Model file for the job. Use its own axes, mm. Face numbers are marked on the shaded views. A direction names the side the tool comes from. Round coordinates to 2 decimals unless told otherwise and drop trailing zeros. Loops run counter-clockwise (first coordinate to the right, second up) from the corner with the lowest first, then second, coordinate; pieces in that order, holes last. Notation, with made-up numbers: M 0.5,-27 L 29.5,-27 A20 cw 29.5,8 Z; hole C -24,-38.75 d10. An arc over 180 degrees is marked long. Answer in a Markdown table with one row per item.
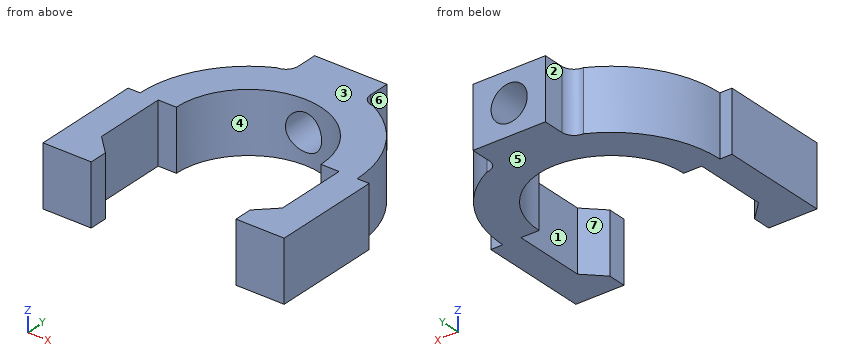
from build123d import *

# Parameters (mm, degrees)
BOSS_EXTRUDE1_DEPTH = 20
SKETCH2_R           = 6
CUT_EXTRUDE1_DEPTH  = 20


with BuildPart() as part:
    # Sketch1 → Boss-Extrude1 (new body)
    with BuildSketch(Plane.XY):
        with BuildLine():
            Line((0, 0), (0, -7))
            ThreePointArc((0, -7), (-1.171572875, -9.828427125), (-4, -11))
            ThreePointArc((-4, -11), (-18.594117082, -24.275365032), (-24, -43.249030993))
            Line((-24, -43.249030993), (-28, -43.249030993))
            Line((-28, -43.249030993), (-28, -79.249030993))
            Line((-28, -79.249030993), (-12, -79.249030993))
            Line((-12, -79.249030993), (-12, -73.249030993))
            Line((-12, -73.249030993), (-18, -67.249030993))
            Line((-18, -67.249030993), (-18, -43.249030993))
            Line((-18, -43.249030993), (-12, -43.249030993))
            ThreePointArc((-12, -43.249030993), (12, -19.249030993), (36, -43.249030993))
            Line((36, -43.249030993), (42, -43.249030993))
            Line((42, -43.249030993), (42, -67.249030993))
            Line((42, -67.249030993), (36, -73.249030993))
            Line((36, -73.249030993), (36, -79.249030993))
            Line((36, -79.249030993), (52, -79.249030993))
            Line((52, -79.249030993), (52, -43.249030993))
            Line((52, -43.249030993), (48, -43.249030993))
            ThreePointArc((48, -43.249030993), (42.594117082, -24.275365032), (28, -11))
            ThreePointArc((28, -11), (25.171572875, -9.828427125), (24, -7))
            Line((24, -7), (24, 0))
            Line((24, 0), (0, 0))
        make_face()
    extrude(amount=BOSS_EXTRUDE1_DEPTH)

    # Sketch2 → Cut-Extrude1 (cut)
    with BuildSketch(Plane(origin=(0, 0, 0), x_dir=(1, 0, 0), z_dir=(0, 1, 0))):
        with Locations((12, -10)):
            Circle(SKETCH2_R)
    extrude(amount=-CUT_EXTRUDE1_DEPTH, mode=Mode.SUBTRACT)


solid = part.part
1. Saw through at B-B (x = 12). Write the cut outline in (y, z), and give its area (3 significant figures).
Verdict:
| item | result |
|---|---|
| outline | M -19.25,0 L 0,0 L 0,4 L -19.25,4 Z; M -19.25,16 L 0,16 L 0,20 L -19.25,20 Z |
| area | 154 mm² |
2. Saw through at C-C (y = -17). Write the cut outline in (x, z).
Verdict:
| item | result |
|---|---|
| outline | M -12.64,0 L 36.64,0 L 36.64,20 L -12.64,20 Z; hole C 12,10 d12 |
3. Mould opens along X. For the marked faces 1, 2, 3 and 4 say: +X half, -X half, draft (parallel to the pull), parting line (faces both ways), or undercut.
Verdict:
| item | result |
|---|---|
| face 1 | undercut |
| face 2 | -X half |
| face 3 | draft |
| face 4 | undercut |
4. Tool access for the marked faces 5, 6 and 7: list every direction of +Z, -Z, +X, -X, +Y, -Y with a clear straight run to the whole face (end or side of a thin tool).
Verdict:
| item | result |
|---|---|
| face 5 | -Z, +X, -X, +Y, -Y |
| face 6 | +Z, -Z, +X, +Y |
| face 7 | +Z, -Z |
5. Saw through at D-D (x = 4). Write the cut outline in (y, z).
Verdict:
| item | result |
|---|---|
| outline | M -20.62,0 L 0,0 L 0,20 L -20.62,20 Z |
6. Wall check: probe 1 along Z at (x, y) = (12, -6); probe 2 along X at (y, z) = (-67, 2); probe 3 along X at (y, z) = (-4.5, 10). Give the ranges that are in metal, low to high.
Verdict:
| item | result |
|---|---|
| probe 1 | z = 0 to 4, 16 to 20 |
| probe 2 | x = -28 to -18, 42 to 52 |
| probe 3 | x = 0 to 6, 18 to 24 |
7. Saw through at A-A (y = -63.5). Write the cut outline in (x, z).
Verdict:
| item | result |
|---|---|
| outline | M -28,0 L -18,0 L -18,20 L -28,20 Z; M 42,0 L 52,0 L 52,20 L 42,20 Z |
8. Pin check, flat tips, straight feed: pin 1 (2 mm diameter, centred on y = -32.5, z = 17.5, fed in from -X); pin 2 (7.5 mm diameter, centred on y = -3.5, z = 5, fed in from +X); pin 3 (1.2 mm diameter, centred on x = 50.5, z = 9.5, fed in from +Y). Stop position of each tip, or through.
Verdict:
| item | result |
|---|---|
| pin 1 | stops at x = -22.65 |
| pin 2 | stops at x = 24.01 |
| pin 3 | stops at y = -43.25 |
